The figure shows three views and two pictorial views of one solid part (mm, origin at its lowest corner). Answer the questions. A direction names the side the tool comes from. Give positions to 0.01 mm unless a question says otherwise; leave off trailing zeros. Loops run counter-clockwise (first coordinate to the right, second up) from the corner with the lowest first, then second, coordinate; pieces in that order, holes last. Notation, with made-up numbers: (0, -10) - (23, -10) arc R19 ccw to (23, 18) - close; hole circle Ø10 at (-2, -3.5). An arc over 180 degrees is marked (long way). Use a Markdown table: item, result. Add a question column.
Item 1: A cutting plane is placed at A-A (x = 22.95). Determine the outline of the cut face in (y, z), plus the area to 3 significant figures.
Item 2: Which of the six approach directions +Z, -Z, +X, -X, +Y, -Y give full straight-line access (tool end or side, diameter ignored) to the marked faces 1, 2 and 3?
Item 3: A cutting plane is placed at D-D (x = 10.75). Determine the outline of the cut face in (y, z), plus the area to 3 significant figures.
Item 4: Each of these flat-tipped pins is pushed along its axis until it touches: P1, Ø7, axis at x = 18, y = 14, coming from the +Z side; P2, Ø0.9, axis at x = 22.5, z = 1.5, coming from the +Y side; P3, Ø2, axis at x = 13, z = 7.5, coming from the +Y side. Where does it stop, or does it pass through?
Item 5: For a pull along Y with two mould halves and no side action, classify the marked faces 4, 5 and 6 as +Y half, -Y half, draft (parallel to the pull), parting line (faces both ways), or undercut.
Item 6: A cutting plane is placed at C-C (z = 2). Determine the outline of the cut face in (x, y), plus the area to 3 significant figures.
Item 7: A cutting plane is placed at B-B (y = 18.25). Determine the outline of the cut face in (x, z), plus the area to 3 significant figures.
Item 8: Consider probe 1 along Y at (x, z) = (10.75, 1.15); probe 2 along X at (y, z) = (21.5, 2) (1 decimal); probe 3 along X at (y, z) = (21, 1.5) (1 decimal). Determine where each line is inside the solid, lowest interval first. Write a range as [from, to].
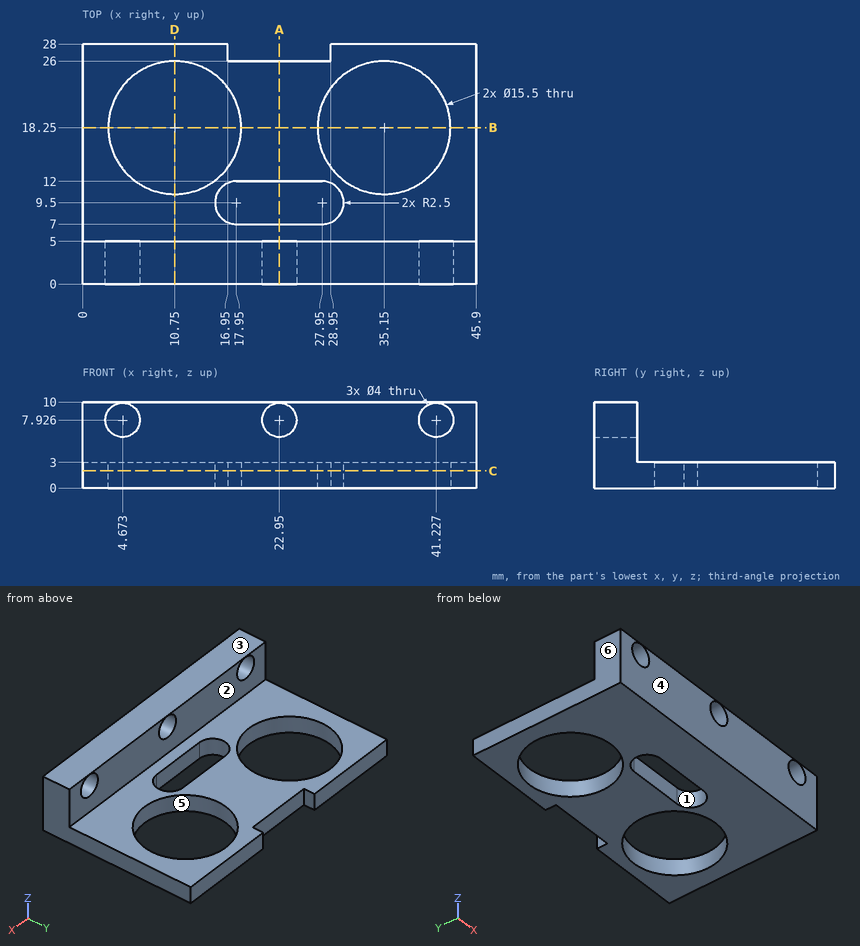
Geometry says:
| question | item | result |
|---|---|---|
| 1 | outline | (0, 0) - (7, 0) - (7, 3) - (5, 3) - (5, 5.93) - (0, 5.93) - close; (0, 9.93) - (5, 9.93) - (5, 10) - (0, 10) - close; (12, 0) - (26, 0) - (26, 3) - (12, 3) - close |
| 1 | area | 78.0 mm² |
| 2 | face 1 | +Z, -Z |
| 2 | face 2 | +Z, +X, -X, +Y |
| 2 | face 3 | +Z, +X, -X, +Y, -Y |
| 3 | outline | (0, 0) - (10.5, 0) - (10.5, 3) - (5, 3) - (5, 10) - (0, 10) - close; (26, 0) - (28, 0) - (28, 3) - (26, 3) - close |
| 3 | area | 72.5 mm² |
| 4 | P1 | z = 3 |
| 4 | P2 | y = 26 |
| 4 | P3 | y = 5 |
| 5 | face 4 | -Y half |
| 5 | face 5 | undercut |
| 5 | face 6 | draft |
| 6 | outline | (0, 0) - (45.9, 0) - (45.9, 28) - (28.95, 28) - (28.95, 26) - (16.95, 26) - (16.95, 28) - (0, 28) - close; hole circle Ø15.5 at (10.75, 18.25); hole (17.95, 7) - (27.95, 7) arc R2.5 ccw to (27.95, 12) - (17.95, 12) arc R2.5 ccw to start; hole circle Ø15.5 at (35.15, 18.25) |
| 6 | area | 814 mm² |
| 7 | outline | (0, 0) - (3, 0) - (3, 3) - (0, 3) - close; (18.5, 0) - (27.4, 0) - (27.4, 3) - (18.5, 3) - close; (42.9, 0) - (45.9, 0) - (45.9, 3) - (42.9, 3) - close |
| 7 | area | 44.7 mm² |
| 8 | probe 1 | [0, 10.5], [26, 28] |
| 8 | probe 2 | [0, 3.7], [17.8, 28.1], [42.2, 45.9] |
| 8 | probe 3 | [0, 3.5], [18, 27.9], [42.4, 45.9] |
